Read the model definition and answer for the solid it produces. Units are mm, in the model's axes. A direction names the side the tool comes from. Give positions to 0.01 mm unless a question says otherwise; leave off trailing zeros. Use a Markdown table: item, result. Add a question column.
Item 1: Consider probe 1 along X at (y, z) = (4.5, 9.5); probe 2 along Y at (x, z) = (31, 3.5); probe 3 along Y at (x, z) = (59, 2). Determine where each line is inside the solid, lowest interval first. Write a range as [from, to].
Item 2: For a pull along X with two mould halves and no side action, classify faces 4 (the face through (113.769, -58.613, 4.93)), 5 (the face through (75.77, -4.8, 4.93)), 6 (the face through (65, 0, 5)) as +X half, -X half, draft (parallel to the pull), parting line (faces both ways), or undercut.
Item 3: Each of these flat-tipped pins is pushed along its axis until it touches: P1, Ø1, axis at x = 57, z = 4.5, coming from the -Y side; P2, Ø4, axis at y = -74.5, z = 3.5, coming from the +X side; P3, Ø5, axis at x = 4.5, z = 3, coming from the +Y side. Where does it stop, or does it pass through?
Item 4: Which of the six approach directions +Z, -Z, +X, -X, +Y, -Y give full straight-line access (tool end or side, diameter ignored) to faces 1 (the face through (88.9, -27.54, 4.93)), 2 (the face through (15, 5, 5)), 3 (the face through (58, 5, 5))?
from build123d import *

# Parameters (mm, degrees)
BOSS_EXTRUDE1_DEPTH = 10
FILLET1_R           = 15


with BuildPart() as part:
    # Sketch1 → Boss-Extrude1 (new body)
    with BuildSketch(Plane.XY):
        with BuildLine():
            Line((0, 0), (15, 0))
            Line((15, 0), (15, 10))
            Line((15, 10), (29, 10))
            Line((29, 10), (29, 0))
            Line((29, 0), (44, 0))
            Line((44, 0), (44, 10))
            Line((44, 10), (58, 10))
            Line((58, 10), (58, 0))
            Line((58, 0), (73, 0))
            Line((73, 0), (78.625, -9.742785793))
            Line((78.625, -9.742785793), (83.821152423, -6.742785793))
            Line((83.821152423, -6.742785793), (91.321152423, -19.733166849))
            Line((91.321152423, -19.733166849), (86.125, -22.733166849))
            Line((86.125, -22.733166849), (91.75, -32.475952642))
            Line((91.75, -32.475952642), (96.946152423, -29.475952642))
            Line((96.946152423, -29.475952642), (104.446152423, -42.466333699))
            Line((104.446152423, -42.466333699), (99.25, -45.466333699))
            Line((99.25, -45.466333699), (104.875, -55.209119491))
            Line((104.875, -55.209119491), (110.071152423, -52.209119491))
            Line((110.071152423, -52.209119491), (117.571152423, -65.199500548))
            Line((117.571152423, -65.199500548), (112.375, -68.199500548))
            Line((112.375, -68.199500548), (118, -77.942286341))
            Line((118, -77.942286341), (87.689110868, -95.442286341))
            add(Edge.make_bspline(
                [(87.689110868, -95.442286341), (77.660181341, -75.620017272), (64.817303381, -57.569676854), (49.160476986, -41.291265088)],
                knots=[0, 0, 0, 0, 1, 1, 1, 1], degree=3))
            add(Edge.make_bspline(
                [(0, -25), (17.242534467, -24.639573707), (35.899987596, -27.504326339), (49.160476986, -41.291265088)],
                knots=[0, 0, 0, 0, 1, 1, 1, 1], degree=3))
            Line((0, -25), (0, 0))
        make_face()
    extrude(amount=BOSS_EXTRUDE1_DEPTH)

    # Fillet1
    fillet1_edges = [part.edges().sort_by_distance(p)[0] for p in [
        (87.689110868, -95.442286341, 5),
        (0, -25, 5),
    ]]
    fillet(fillet1_edges, radius=FILLET1_R)


solid = part.part
Geometry says:
| question | item | result |
|---|---|---|
| 1 | probe 1 | [15, 29], [44, 58] |
| 1 | probe 2 | [-29.46, 0] |
| 1 | probe 3 | [-52.19, 0] |
| 2 | face 4 | +X half |
| 2 | face 5 | undercut |
| 2 | face 6 | draft |
| 3 | P1 | y = -50.44 |
| 3 | P2 | x = 117.17 |
| 3 | P3 | y = 0 |
| 4 | face 1 | +Z, -Z |
| 4 | face 2 | +Z, -Z, -X, +Y |
| 4 | face 3 | +Z, -Z, +X, +Y |
